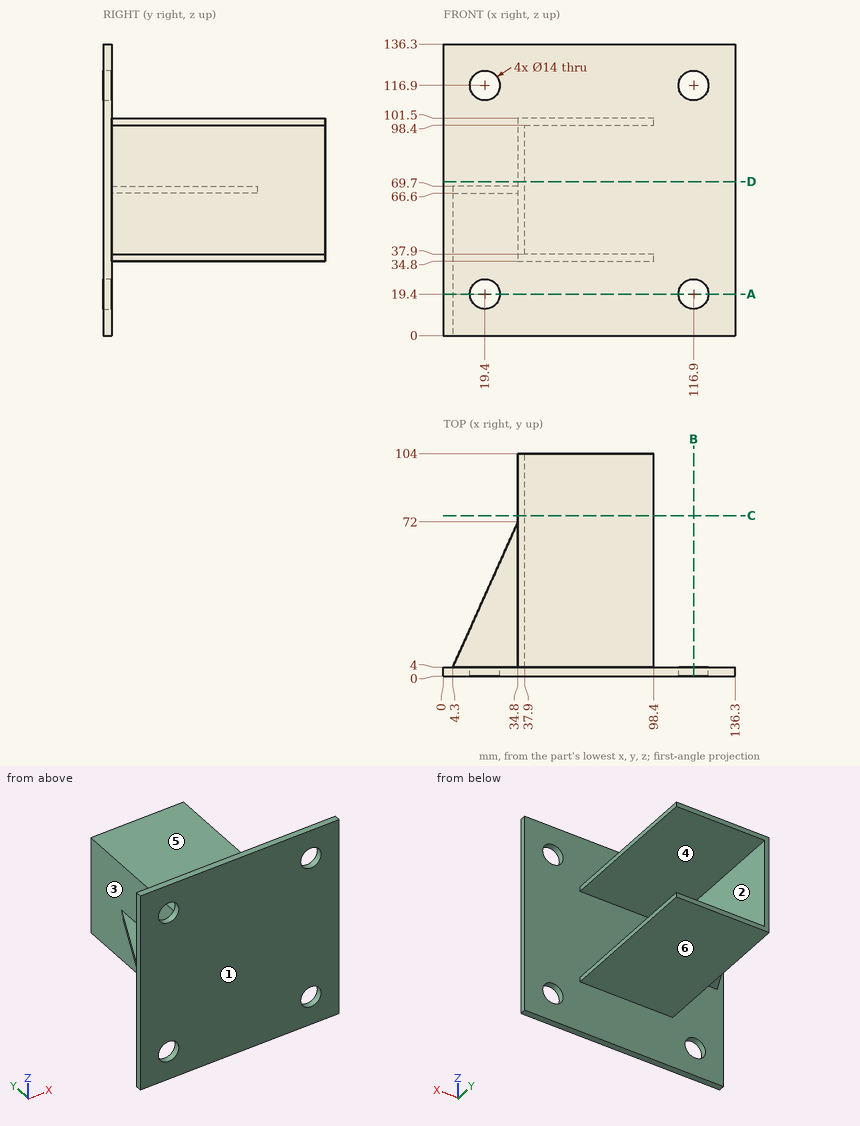
Check sheet for the drawn part. Datum: minimum x, y, z corner. Units: mm. A direction names the side the tool comes from. Give positions to 0.01 mm unless a question says otherwise; leave off trailing zeros. Order: outer loops, then holes, each group sorted by start corner. A loop starts at its lowest first (then second) coordinate and runs counter-clockwise, first axis right, second up. Notation, with made-up numbers: (-15, 36.5) -> (14, 36.5) arc R34 cw to (14, 69.5) -> close; hole circle Ø10 at (53, 6). An arc over 180 degrees is marked (long way). Use a Markdown table: item, result.
1) Depth check by flat-ended pin: pin 1 Ø0.9 at (y, z) = (53.5, 100.5) entering from +X; pin 2 Ø2 at (y, z) = (42, 78) entering from +X; pin 3 Ø9 at (x, y) = (21, 52) entering from +Z. Enter the tip coordinate at first touch or a pass-through.
Results:
| item | result |
|---|---|
| pin 1 | x = 98.4 |
| pin 2 | x = 37.9 |
| pin 3 | z = 69.7 |
2) Tool access check on the marked faces 1, 2 and 3. Record the directions out of +Z, -Z, +X, -X, +Y, -Y that give a thin tool (end or side, any length) a straight path to the whole face; none if there is none.
Results:
| item | result |
|---|---|
| face 1 | +Z, -Z, +X, -X, -Y |
| face 2 | +X, +Y |
| face 3 | -X, +Y |
3) Section check B-B, the plane x = 116.9. Record the boundary of the cut face in (y, z), then the cut area to 3 significant figures.
Results:
| item | result |
|---|---|
| outline | (0, 0) -> (4, 0) -> (4, 12.4) -> (0, 12.4) -> close; (0, 26.4) -> (4, 26.4) -> (4, 109.9) -> (0, 109.9) -> close; (0, 123.9) -> (4, 123.9) -> (4, 136.3) -> (0, 136.3) -> close |
| area | 433 mm² |
4) Section check D-D, the plane z = 72. Record the boundary of the cut face in (x, y), then the cut area to 3 significant figures.
Results:
| item | result |
|---|---|
| outline | (0, 0) -> (136.3, 0) -> (136.3, 4) -> (37.9, 4) -> (37.9, 104) -> (34.8, 104) -> (34.8, 4) -> (0, 4) -> close |
| area | 855 mm² |
5) Section check A-A, the plane z = 19.4. Record the boundary of the cut face in (x, y), then the cut area to 3 significant figures.
Results:
| item | result |
|---|---|
| outline | (0, 0) -> (12.4, 0) -> (12.4, 4) -> (0, 4) -> close; (26.4, 0) -> (109.9, 0) -> (109.9, 4) -> (26.4, 4) -> close; (123.9, 0) -> (136.3, 0) -> (136.3, 4) -> (123.9, 4) -> close |
| area | 433 mm² |
6) Material ranges on probe 1 along X at (y, z) = (1, 19.4); probe 2 along Z at (x, y) = (65.5, 45); probe 3 along X at (y, z) = (2, 116), recorded low to high.
Results:
| item | result |
|---|---|
| probe 1 | 0 to 12.4, 26.4 to 109.9, 123.9 to 136.3 |
| probe 2 | 34.8 to 37.9, 98.4 to 101.5 |
| probe 3 | 0 to 12.46, 26.34 to 109.96, 123.84 to 136.3 |
7) Section check C-C, the plane y = 75. Record the boundary of the cut face in (x, z).
Results:
| item | result |
|---|---|
| outline | (34.8, 34.8) -> (98.4, 34.8) -> (98.4, 37.9) -> (37.9, 37.9) -> (37.9, 98.4) -> (98.4, 98.4) -> (98.4, 101.5) -> (34.8, 101.5) -> close |
8) Mould release check, pull along Z, two halves, no side actions. Record for the marked faces 4, 5 and 6: pulls with the +Z half, pulls with the -Z half, needs draft (parallel to the pull), parting line crosses it, or undercut.
Results:
| item | result |
|---|---|
| face 4 | undercut |
| face 5 | pulls with the +Z half |
| face 6 | pulls with the -Z half |
